Autodesk Inventor part; units mm, degrees
ref_plane "YZ Plane" through (0, 0, 0) normal (1, 0, 0) x (0, 1, 0)
ref_plane "XZ Plane" through (0, 0, 0) normal (0, 1, 0) x (-1, 0, 0)
ref_plane "XY Plane" through (0, 0, 0) normal (0, 0, 1) x (1, 0, 0)
sketch "Sketch1" plane through (0, 0, 0) normal (1, 0, 0) x (0, 1, 0)
  line L0 (0, 0) -> (0, 152.4)
  line L1 (0, 0) -> (330.2, 0)
  line L2 (0, 152.4) -> (342.9, 152.4)
  line L3 (342.9, 152.4) -> (342.9, 139.7) construction
  arc A0 (355.3918, 137.4098) -> (342.9, 152.4) centre (342.9, 139.7) ccw
  line L4 (330.2, 0) -> (355.7981, 139.6261)
  dimension "d0" = 152.4
  dimension "d1" = 330.2
  dimension "d2" = 342.9
  dimension "d3" = 12.7
extrude "Extrusion1" add sketch "Sketch1" along normal blind 1249.5609
properties part number "D" material "Granite, Cut, Polished"
Work out the finished part from the listing and answer in its coordinate system (mm). Coordinates: 2 decimals unless noted, no trailing zeros. Write each loop counter-clockwise with the first axis right and the second up, starting at its lowest first coordinate (ties: lowest second). Pieces come first, ordered by that corner, then holes.
Q1. Each of these flat-tipped pins is pushed along its axis until it touches: pin 1 Ø3 at (x, z) = (430, 67.5) entering from +Y; pin 2 Ø6 at (x, z) = (130.5, 116) entering from +Y. Where does it stop, or does it pass through?
Q2. A cutting plane is placed at B-B, the plane z = 12. Give the vertices of the cut face in (x, y).
Q3. A cutting plane is placed at C-C, the plane z = 62. Give the vertices of the cut face in (x, y), then the cut area to 3 significant figures.
Q4. A cutting plane is placed at A-A, the plane x = 921.5. Give the vertices of the cut face in (y, z).
Q5. Find the intervals of material crossed by line 1 (Y direction, x = 642, z = 142); line 2 (Y direction, x = 60.5, z = 140.5), in increasing order.
Findings below:
1. pin 1: stops at y = 342.85
1. pin 2: stops at y = 352.02
2. outline: (0, 0) - (1249.56, 0) - (1249.56, 332.4) - (0, 332.4) - close
3. outline: (0, 0) - (1249.56, 0) - (1249.56, 341.57) - (0, 341.57) - close
3. area: 427,000 mm2
4. outline: (0, 0) - (330.2, 0) - (355.39, 137.41) arc R12.7 ccw to (342.9, 152.4) - (0, 152.4) - close
5. line 1: y = 0 to 355.39
5. line 2: y = 0 to 355.57
